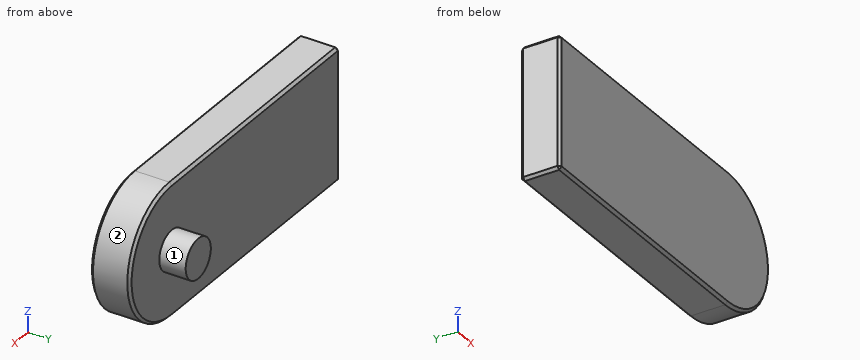
from build123d import *

# Parameters (mm, degrees)
BOSS_EXTRUDE1_DEPTH = 30
SKETCH2_R           = 15
BOSS_EXTRUDE2_DEPTH = 20
CHAMFER1_SIZE       = 2


with BuildPart() as part:
    # Sketch1 → Boss-Extrude1 (new body)
    with BuildSketch(Plane(origin=(0, 0, 0), x_dir=(1, 0, 0), z_dir=(0, 1, 0))):
        with BuildLine():
            Line((100, 50), (-100, 50))
            Line((-100, 50), (-100, -50))
            Line((-100, -50), (100, -50))
            ThreePointArc((100, -50), (150, 0), (100, 50))
        make_face()
    extrude(amount=BOSS_EXTRUDE1_DEPTH)

    # Sketch2 → Boss-Extrude2 (add)
    with BuildSketch(Plane(origin=(0, 30, 0), x_dir=(1, 0, 0), z_dir=(0, 1, 0))):
        with Locations((100, 0)):
            Circle(SKETCH2_R)
    extrude(amount=BOSS_EXTRUDE2_DEPTH)

    # Chamfer1
    chamfer1_edges = [part.edges().sort_by_distance(p)[0] for p in [
        (-100, 30, 0),
        (0, 30, 50),
        (150, 30, 0),
        (0, 0, 50),
        (-100, 0, 0),
        (0, 0, -50),
        (150, 0, 0),
        (-100, 15, 50),
        (-100, 15, -50),
        (0, 30, -50),
    ]]
    chamfer(chamfer1_edges, length=CHAMFER1_SIZE)


solid = part.part
Source: CAD feature listing. Evaluate the final solid. Frame: model axes, mm. Face numbers are marked on the shaded views. A direction names the side the tool comes from. Give positions to 0.01 mm unless a question says otherwise; leave off trailing zeros. Order: outer loops, then holes, each group sorted by start corner. A loop starts at its lowest first (then second) coordinate and runs counter-clockwise, first axis right, second up. Notation, with made-up numbers: (43.5, 79) -> (81.5, 79) arc R29 cw to (81.5, 112) -> close; hole circle Ø11 at (-23, 20.25). An arc over 180 degrees is marked (long way). Write item = value, one per line.
Q1. Pin query (flat end, axial travel): pin 1 (1.5 mm diameter, centred on x = 25, z = -26.5, fed in from +Y); pin 2 (4 mm diameter, centred on y = 17.5, z = -23.5, fed in from +X); pin 3 (5 mm diameter, centred on x = 57.5, y = 32, fed in from +Z). Return the tip coordinate at first contact, or that it passes through.
Data:
pin_1 = 30
pin_2 = 145.14
pin_3 = 48.5
Q2. Cut plane B-B, the plane y = 18.5. Output: boundary loops of the cut face in (x, z).
Data:
outline = (-100, -48) -> (-98, -50) -> (100, -50) arc R50 ccw to (100, 50) -> (-98, 50) -> (-100, 48) -> close
Q3. Material intervals for line 1 (Y direction, x = 101, z = 40.5); line 2 (X direction, y = 24, z = 2); line 3 (X direction, y = 37, z = 0.5), sorted ascending. Write a range as from..to.
Data:
line_1 = 0..30
line_2 = -100..149.96
line_3 = 85.01..114.99
Q4. Cut plane A-A, the plane z = 0. Output: boundary loops of the cut face in (x, y), and give its area (3 significant figures).
Data:
outline = (-100, 2) -> (-98, 0) -> (148, 0) -> (150, 2) -> (150, 28) -> (148, 30) -> (115, 30) -> (115, 50) -> (85, 50) -> (85, 30) -> (-98, 30) -> (-100, 28) -> close
area = 8,090 mm^2
Q5. Cut plane D-D, the plane y = 38. Output: boundary loops of the cut face in (x, z), and give its area (3 significant figures).
Data:
outline = circle Ø30 at (100, 0)
area = 707 mm^2
Q6. Set-up query: the marked faces 1 and 2. Return all of +Z, -Z, +X, -X, +Y, -Y with unobstructed straight access to the full face (end or side cutting, diameter ignored); none if empty.
Data:
face_1 = +Y
face_2 = +X, +Y, -Y
Q7. Cut plane C-C, the plane x = 91.5. Output: boundary loops of the cut face in (y, z), and give its area (3 significant figures).
Data:
outline = (0, -48) -> (2, -50) -> (28, -50) -> (30, -48) -> (30, -12.36) -> (50, -12.36) -> (50, 12.36) -> (30, 12.36) -> (30, 48) -> (28, 50) -> (2, 50) -> (0, 48) -> close
area = 3,490 mm^2
